from build123d import *

# Parameters (mm, degrees)
F0_R     = 6.35
F1_DEPTH = 12


with BuildPart() as f1:
    # F0 (on Top) → F1 (new body)
    with BuildSketch(Plane.XY):
        with Locations((0, 0.103021)):
            Circle(F0_R)
        with BuildLine():
            ThreePointArc((-2.645654, -0.64732), (-2.75, 0.103021), (-2.645654, 0.853363))
            Line((-2.645654, 0.853363), (-3.800122, 1.180785))
            ThreePointArc((-3.800122, 1.180785), (-3.4208, 2.078021), (-2.833431, 2.855142))
            Line((-2.833431, 2.855142), (-1.972642, 2.019054))
            ThreePointArc((-1.972642, 2.019054), (-1.375, 2.484591), (-0.673012, 2.769396))
            Line((-0.673012, 2.769396), (-0.96669, 3.932905))
            ThreePointArc((-0.96669, 3.932905), (0, 4.053021), (0.96669, 3.932905))
            Line((0.96669, 3.932905), (0.673012, 2.769396))
            ThreePointArc((0.673012, 2.769396), (1.375, 2.484591), (1.972642, 2.019054))
            Line((1.972642, 2.019054), (2.833431, 2.855142))
            ThreePointArc((2.833431, 2.855142), (3.4208, 2.078021), (3.800122, 1.180785))
            Line((3.800122, 1.180785), (2.645654, 0.853363))
            ThreePointArc((2.645654, 0.853363), (2.75, 0.103021), (2.645654, -0.64732))
            Line((2.645654, -0.64732), (3.800122, -0.974742))
            ThreePointArc((3.800122, -0.974742), (3.4208, -1.871979), (2.833431, -2.649099))
            Line((2.833431, -2.649099), (1.972642, -1.813012))
            ThreePointArc((1.972642, -1.813012), (1.375, -2.278549), (0.673012, -2.563353))
            Line((0.673012, -2.563353), (0.96669, -3.726862))
            ThreePointArc((0.96669, -3.726862), (0, -3.846979), (-0.96669, -3.726862))
            Line((-0.96669, -3.726862), (-0.673012, -2.563353))
            ThreePointArc((-0.673012, -2.563353), (-1.375, -2.278549), (-1.972642, -1.813012))
            Line((-1.972642, -1.813012), (-2.833431, -2.649099))
            ThreePointArc((-2.833431, -2.649099), (-3.4208, -1.871979), (-3.800122, -0.974742))
            Line((-3.800122, -0.974742), (-2.645654, -0.64732))
        make_face(mode=Mode.SUBTRACT)
    extrude(amount=F1_DEPTH)


solid = f1.part
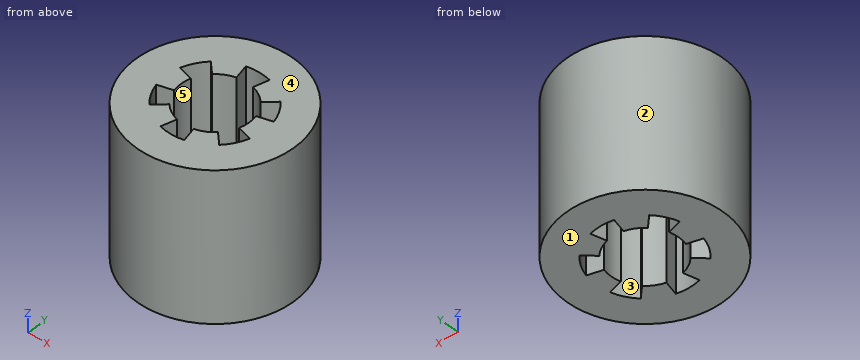
Could you check a few things on this model? Use its own coordinates, in mm. Face numbers are marked on the shaded views. A direction names the side the tool comes from. Give positions to 0.01 mm unless a question says otherwise; leave off trailing zeros. Write each loop counter-clockwise with the first axis right and the second up, starting at its lowest first coordinate (ties: lowest second). Pieces come first, ordered by that corner, then holes. Notation, with made-up numbers: (3.25, -38) -> (62.25, -38) arc R15 cw to (62.25, -15) -> close; hole circle Ø7 at (71, 19.5). An arc over 180 degrees is marked (long way). Answer as a JSON object with one key per item and string values.
Q1. Suppose I cut it at B-B on z = 7. Write out the boundary of the cut face in (x, y), then the cut area to 3 significant figures.
Taken from the geometry:
{"outline": "circle Ø12.7 at (0, 0.1); hole (-3.8, -0.97) arc R3.95 ccw to (-2.83, -2.65) -> (-1.97, -1.81) arc R2.75 ccw to (-0.67, -2.56) -> (-0.97, -3.73) arc R3.95 ccw to (0.97, -3.73) -> (0.67, -2.56) arc R2.75 ccw to (1.97, -1.81) -> (2.83, -2.65) arc R3.95 ccw to (3.8, -0.97) -> (2.65, -0.65) arc R2.75 ccw to (2.65, 0.85) -> (3.8, 1.18) arc R3.95 ccw to (2.83, 2.86) -> (1.97, 2.02) arc R2.75 ccw to (0.67, 2.77) -> (0.97, 3.93) arc R3.95 ccw to (-0.97, 3.93) -> (-0.67, 2.77) arc R2.75 ccw to (-1.97, 2.02) -> (-2.83, 2.86) arc R3.95 ccw to (-3.8, 1.18) -> (-2.65, 0.85) arc R2.75 ccw to (-2.65, -0.65) -> close", "area": "91.0 mm²"}
Q2. Suppose I cut it at C-C on x = 1.75. Write out the boundary of the cut face in (y, z).
Taken from the geometry:
{"outline": "(-6, 0) -> (-2.02, 0) -> (-2.02, 12) -> (-6, 12) -> close; (2.22, 0) -> (6.21, 0) -> (6.21, 12) -> (2.22, 12) -> close"}
Q3. Will these pins go through, and if not, where does the flat tip stop? pin 1 Ø6 at (x, z) = (3.5, 10) entering from -Y; pin 2 Ø1 at (x, z) = (-3, 5.5) entering from -Y.
Taken from the geometry:
{"pin 1": "stops at y = -6.23", "pin 2": "stops at y = -5.73"}
Q4. Suppose I cut it at A-A on x = 0. Write out the boundary of the cut face in (y, z).
Taken from the geometry:
{"outline": "(-6.25, 0) -> (-3.85, 0) -> (-3.85, 12) -> (-6.25, 12) -> close; (4.05, 0) -> (6.45, 0) -> (6.45, 12) -> (4.05, 12) -> close"}
Q5. Suppose I cut it at D-D on y = 4.75. Write out the boundary of the cut face in (x, z).
Taken from the geometry:
{"outline": "(-4.33, 0) -> (4.33, 0) -> (4.33, 12) -> (-4.33, 12) -> close"}
Q6. We'd pull the mould along Y, two halves only. Please class the marked faces 1, 2 and 3: released by +Y, released by -Y, zero draft, split by the parting line, or undercut.
Taken from the geometry:
{"face 1": "zero draft", "face 2": "split by the parting line", "face 3": "undercut"}
Q7. Please list where these lines run through material, in increasing order: L1, parallel to Y at x = 3.5, z = 1.75; L2, parallel to X at y = 2.5, z = 0.75; L3, parallel to Y at x = -3.25, z = 7.
Taken from the geometry:
{"L1": "y = -5.2 to -1.73, -0.89 to 1.1, 1.93 to 5.4", "L2": "x = -5.88 to -3.14, -2.47 to -1.35, 1.35 to 2.47, 3.14 to 5.88", "L3": "y = -5.35 to -2.14, -0.82 to 1.02, 2.35 to 5.56"}
Q8. Which directions (+Z, -Z, +X, -X, +Y, -Y) give clear straight access to the entire face, cutting with the end or side of a thin tool? Please do the marked faces 4 and 5.
Taken from the geometry:
{"face 4": "+Z, +X, -X, +Y, -Y", "face 5": "+Z, -Z"}
